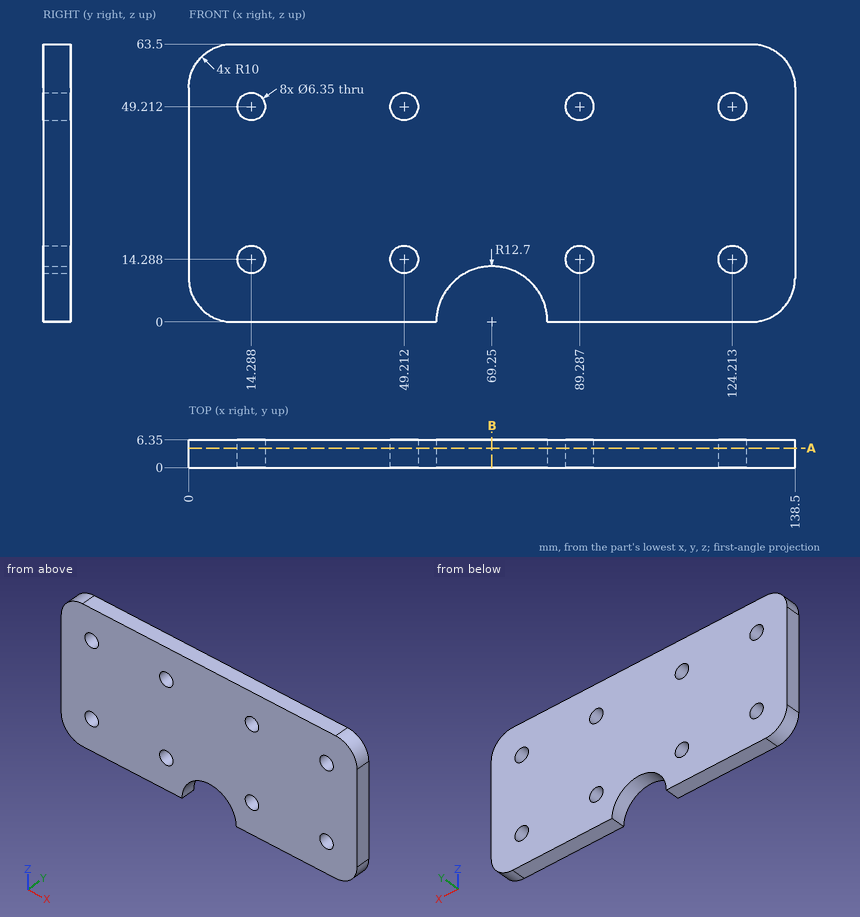
Drawing for the job (mm, zero at the part's lowest x, y, z). Coordinates: 2 decimals unless noted, no trailing zeros. Write each loop counter-clockwise with the first axis right and the second up, starting at its lowest first coordinate (ties: lowest second). Pieces come first, ordered by that corner, then holes. Notation, with made-up numbers: (21.25, 81) - (35.25, 81) arc R25 ccw to (35.25, 102) - close; hole circle Ø6 at (25, 65.25). An arc over 180 degrees is marked (long way). Write each question's results on one line, items separated by ' | '. Start each with the question number.
1) Cut at B-B (x = 69.25). Write the cut outline in (y, z).
2) Flat gauge pin, fed straight in: P1, Ø5.5, axis at x = 14.29, z = 14.29, coming from the +Y side. Where does the tip first touch, or does it go through?
3) Probe line 1 along Z through (x, y) = (122.5, 2) (1 decimal); line 2 along Z through (x, y) = (15, 2.75); line 3 along Z through (x, y) = (8.5, 2.25). List the from-to ranges inside material, lowest first. Write a range as from..to.
4) Cut at A-A (y = 4.5). Count the separate pieces of the cut face and the enclosed holes in it, then the cut area to 3 significant figures.
Returned:
1) outline: (0, 12.7) - (6.35, 12.7) - (6.35, 63.5) - (0, 63.5) - close
2) P1: through
3) line 1: 0..11.6, 17..46.5, 51.9..63.5 | line 2: 0..11.19, 17.38..46.12, 52.31..63.5 | line 3: 0.11..63.39
4) separate pieces: 1 | enclosed holes: 8 | area: 8,200 mm^2
